For this review, take the finished solid that the model builds, in its own axes (mm). A direction names the side the tool comes from. Coordinates: 2 decimals unless noted, no trailing zeros. Order: outer loops, then holes, each group sorted by start corner. A loop starts at its lowest first (then second) coordinate and runs counter-clockwise, first axis right, second up. Notation, with made-up numbers: M 61.5,-26.5 L 78.5,-26.5 A15 cw 78.5,-19.5 Z; hole C 51,33.25 d8. An arc over 180 degrees is marked long. Use one line per item in the form item = value. Start each with the question number.
```python
from build123d import *

# Parameters (mm, degrees)
EXTRUDE_1_DEPTH = 150
EXTRUDE_2_DEPTH = 50
SKETCH_4_R      = 25
EXTRUDE_3_DEPTH = 80
SKETCH_5_W      = 60
SKETCH_5_H      = 60
EXTRUDE_4_DEPTH = 53
SKETCH_6_R      = 10
EXTRUDE_5_DEPTH = 15
SKETCH_7_R      = 20
EXTRUDE_6_DEPTH = 12
SKETCH_8_R      = 4.914054778
EXTRUDE_7_DEPTH = 22


with BuildPart() as part:
    # ｽｹｯﾁ1 → ﾎﾞｽ - 押し出し1 (new body)
    with BuildSketch(Plane.XY):
        Polygon((0, 0), (120, 0), (120, 240), (70, 240), (70, 40), (0, 40), align=None)
    extrude(amount=EXTRUDE_1_DEPTH)

    # ｽｹｯﾁ3 → ﾎﾞｽ - 押し出し2 (add)
    with BuildSketch(Plane(origin=(0, 80, 0), x_dir=(1, 0, 0), z_dir=(0, 1, 0))):
        with BuildLine():
            Line((70, -40), (-30, -40))
            ThreePointArc((-30, -40), (-65, -75), (-30, -110))
            Line((-30, -110), (70, -110))
            Line((70, -110), (70, -40))
        make_face()
    extrude(amount=EXTRUDE_2_DEPTH)

    # ｽｹｯﾁ4 → ﾎﾞｽ - 押し出し3 (add)
    with BuildSketch(Plane(origin=(0, 130, 0), x_dir=(1, 0, 0), z_dir=(0, 1, 0))):
        with Locations((-29.999997022, -75)):
            Circle(SKETCH_4_R)
    extrude(amount=EXTRUDE_3_DEPTH)

    # ｽｹｯﾁ5 → ﾎﾞｽ - 押し出し4 (add)
    with BuildSketch(Plane(origin=(0, 240, 0), x_dir=(1, 0, 0), z_dir=(0, 1, 0))):
        with Locations((95, -75)):
            Rectangle(SKETCH_5_W, SKETCH_5_H)
    extrude(amount=EXTRUDE_4_DEPTH)

    # ｽｹｯﾁ6 → ﾎﾞｽ - 押し出し5 (add)
    with BuildSketch(Plane(origin=(0, 293, 0), x_dir=(1, 0, 0), z_dir=(0, 1, 0))):
        with Locations((95, -75)):
            Circle(SKETCH_6_R)
    extrude(amount=EXTRUDE_5_DEPTH)

    # ｽｹｯﾁ7 → ﾎﾞｽ - 押し出し6 (add)
    with BuildSketch(Plane(origin=(0, 308, 0), x_dir=(1, 0, 0), z_dir=(0, 1, 0))):
        with Locations((95, -75)):
            Circle(SKETCH_7_R)
    extrude(amount=EXTRUDE_6_DEPTH)

    # ｽｹｯﾁ8 → ﾎﾞｽ - 押し出し7 (add)
    with BuildSketch(Plane(origin=(0, 320, 0), x_dir=(1, 0, 0), z_dir=(0, 1, 0))):
        with Locations((85.328318408, -65.952959142)):
            Circle(SKETCH_8_R)
    extrude(amount=EXTRUDE_7_DEPTH)


solid = part.part
```
1. The part is to be moulded in two halves that separate along Y. For faces 5 (the cylindrical face through (87.63, 300.4, 68.24)), 6 (the flat face through (-30, 210, 75)), 7 (the flat face through (95, 266, 105)), say which applies: pulls with the +Y half, pulls with the -Y half, needs draft (parallel to the pull), parting line crosses it, or undercut.
2. Consider section A-A, the plane y = 171. Write out the cut boundary in (x, z).
3. Tool access review of faces 1 (the flat face through (65, 266, 75)), 2 (the flat face through (95, 240, 127)), 3 (the flat face through (86, 308, 70)), 4 (the flat face through (95, 240, 22)): name each direction out of +Z, -Z, +X, -X, +Y, -Y from which nothing blocks a thin tool from reaching the whole face with its end or side.
4. Consider section D-D, the plane x = 95. Write out the cut boundary in (y, z).
5. Consider section B-B, the plane x = 35. Write out the cut boundary in (y, z).
6. Consider section C-C, the plane z = 75. Write out the cut boundary in (x, y).
7. For pin 1 Ø25 at (x, y) = (44, 102) entering from -Z; pin 2 Ø15 at (x, y) = (15, 94.5) entering from +Z; pin 3 Ø5 at (y, z) = (89.5, 59.5) entering from -X; pin 4 Ø10 at (y, z) = (293.5, 35.5) entering from +X, all flat-tipped, find the tip position at first contact; note any pin that passes through.
8. To check wall thickness, follow line 1 (Y direction, x = 69, z = 83); line 2 (Y direction, x = 43.5, z = 45); line 3 (Y direction, x = 77, z = 75). State the ranges of each line that lie inside material, in increasing order.
Answers follow:
q1.face_5 = undercut
q1.face_6 = pulls with the +Y half
q1.face_7 = needs draft
q2.outline = C -30,75 d50; M 70,0 L 120,0 L 120,150 L 70,150 Z
q3.face_1 = +Z, -Z, -X, +Y
q3.face_2 = +Z, +X, -X, +Y
q3.face_3 = none
q3.face_4 = -Z, +X, -X, +Y
q4.outline = M 0,0 L 240,0 L 240,45 L 293,45 L 293,65 L 308,65 L 308,55 L 320,55 L 320,95 L 308,95 L 308,85 L 293,85 L 293,105 L 240,105 L 240,150 L 0,150 Z
q5.outline = M 0,0 L 40,0 L 40,150 L 0,150 Z; M 80,40 L 130,40 L 130,110 L 80,110 Z
q6.outline = M -65,80 L 70,80 L 70,40 L 0,40 L 0,0 L 120,0 L 120,240 L 125,240 L 125,293 L 105,293 L 105,308 L 115,308 L 115,320 L 75,320 L 75,308 L 85,308 L 85,293 L 65,293 L 65,240 L 70,240 L 70,130 L -5,130 L -5,210 L -55,210 L -55,130 L -65,130 Z
q7.pin_1 = 40
q7.pin_2 = 110
q7.pin_3 = -62.5
q7.pin_4 = through
q8.line_1 = 0 to 40, 80 to 130, 240 to 293
q8.line_2 = 0 to 40, 80 to 130
q8.line_3 = 0 to 293, 308 to 320
